Part model, mm, in its own coordinate system. Face numbers are marked on the shaded views. A direction names the side the tool comes from. Round coordinates to 2 decimals unless told otherwise and drop trailing zeros. Write each loop counter-clockwise with the first axis right and the second up, starting at its lowest first coordinate (ties: lowest second). Pieces come first, ordered by that corner, then holes.
1) Flat gauge pins, fed straight in: pin 1 (12 mm diameter, centred on x = 109.5, y = -37.5, fed in from +Z); pin 2 (1 mm diameter, centred on x = 193.5, z = 236, fed in from +Y). Where does each tip first touch, or does it go through?
2) Saw through at A-A on y = 139. Write the cut outline in (x, z), and give its area (3 significant figures).
3) Saw through at D-D on y = -138.5. Write the cut outline in (x, z).
4) Which spindle directions (+Z, -Z, +X, -X, +Y, -Y) get a long thin tool onto all of the face, cutting with end or side? Do the marked faces 1, 2 and 3. Say none if no direction does.
5) Saw through at C-C on x = -369. Write the cut outline in (y, z), and give its area (3 significant figures).
6) Saw through at B-B on z = 149. Write the cut outline in (x, y), and give its area (3 significant figures).
7) Drill centre lines: L1, parallel to X at y = -108, z = 217; L2, parallel to Y at x = 322, z = 142; L3, parallel to Z at x = 57, y = -154. Where is each one in solid material? Low to high.
```python
from build123d import *

# Parameters (mm, degrees)
F1_DEPTH = 200
F3_DEPTH = 200


with BuildPart() as f1:
    # F0 (on Front) → F1 (new body)
    with BuildSketch(Plane.XZ):
        Polygon((-150, 325), (-450, 325), (-450, -325), (450, -325), (450, 325), (150, 325), (150, 75), (-150, 75), align=None)
    extrude(amount=F1_DEPTH)

    # F2 (on face) → F3 (join)
    with BuildSketch(Plane(origin=(0, 0, 0), x_dir=(-1, 0, 0), z_dir=(0, 1, 0))):
        Polygon((450, -325), (450, 325), (150, -325), align=None)
        Polygon((-150, -325), (-450, 325), (-450, -325), align=None)
    extrude(amount=F3_DEPTH)


solid = f1.part
```
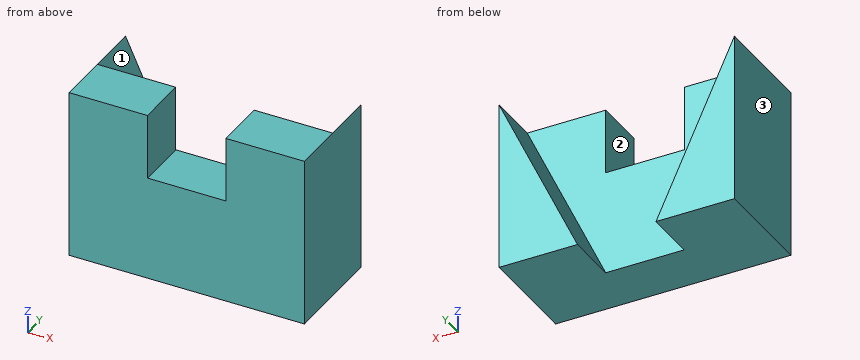
Completed:
1. pin 1: stops at z = 75
1. pin 2: stops at y = 0
2. outline: (-450, -325) - (-150, -325) - (-450, 325) - close; (150, -325) - (450, -325) - (450, 325) - close
2. area: 195,000 mm2
3. outline: (-450, -325) - (450, -325) - (450, 325) - (150, 325) - (150, 75) - (-150, 75) - (-150, 325) - (-450, 325) - close
4. face 1: +Z, +Y
4. face 2: +Z, +Y, -Y
4. face 3: +Z, -Z, -X, +Y, -Y
5. outline: (-200, -325) - (200, -325) - (200, 149.5) - (0, 149.5) - (0, 325) - (-200, 325) - close
5. area: 225,000 mm2
6. outline: (-450, -200) - (-150, -200) - (-150, 0) - (-368.77, 0) - (-368.77, 200) - (-450, 200) - close; (150, -200) - (450, -200) - (450, 200) - (368.77, 200) - (368.77, 0) - (150, 0) - close
6. area: 152,000 mm2
7. L1: x = -450 to -150, 150 to 450
7. L2: y = -200 to 0
7. L3: z = -325 to 75
